```python
from build123d import *

# Parameters (mm, degrees)
BOSS_EXTRUDE1_DEPTH      = 10
BOSS_EXTRUDE1_DEPTH_BACK = 10
FILLET1_R                = 10


with BuildPart() as part:
    # Sketch1 → Boss-Extrude1 (new, two sides: drawn at the far end of the back side and taken through both)
    with BuildSketch(Plane.XY.offset(-BOSS_EXTRUDE1_DEPTH_BACK)):
        with BuildLine():
            Line((237.926881338, -1499.570637215), (237.926881338, -1519.570637215))
            Line((237.926881338, -1519.570637215), (214.725572022, -1519.570637215))
            ThreePointArc((214.725572022, -1519.570637215), (201.473903455, -1517.311772335), (189.718921324, -1510.790301224))
            Line((189.718921324, -1510.790301224), (-403.542618158, -1035.59351223))
            ThreePointArc((-403.542618158, -1035.59351223), (-414.593324739, -1021.690516088), (-418.53596746, -1004.37384822))
            Line((-418.53596746, -1004.37384822), (-418.53596746, -990.945694684))
            Line((-418.53596746, -990.945694684), (-398.53596746, -990.945694684))
            Line((-398.53596746, -990.945694684), (-398.53596746, -1004.37384822))
            ThreePointArc((-398.53596746, -1004.37384822), (-396.5646461, -1013.032182154), (-391.039292809, -1019.983680225))
            Line((-391.039292809, -1019.983680225), (202.222246673, -1495.180469219))
            ThreePointArc((202.222246673, -1495.180469219), (208.099737738, -1498.441204775), (214.725572022, -1499.570637215))
            Line((214.725572022, -1499.570637215), (237.926881338, -1499.570637215))
        make_face()
    extrude(amount=BOSS_EXTRUDE1_DEPTH + BOSS_EXTRUDE1_DEPTH_BACK)

    # Fillet1
    fillet1_edges = [part.edges().sort_by_distance(p)[0] for p in [
        (226.32622668, -1499.570637215, -10),
        (208.099737738, -1498.441204775, -10),
        (-398.53596746, -997.659771452, -10),
        (-396.5646461, -1013.032182154, -10),
        (-418.53596746, -997.659771452, -10),
        (-414.593324739, -1021.690516088, -10),
        (226.32622668, -1519.570637215, -10),
        (201.473903455, -1517.311772335, -10),
        (226.32622668, -1499.570637215, 10),
        (208.099737738, -1498.441204775, 10),
        (-398.53596746, -997.659771452, 10),
        (-396.5646461, -1013.032182154, 10),
        (-418.53596746, -997.659771452, 10),
        (-414.593324739, -1021.690516088, 10),
        (226.32622668, -1519.570637215, 10),
        (201.473903455, -1517.311772335, 10),
        (-94.408523068, -1257.582074722, -10),
        (-106.911848417, -1273.191906727, -10),
        (-94.408523068, -1257.582074722, 10),
        (-106.911848417, -1273.191906727, 10),
    ]]
    fillet(fillet1_edges, radius=FILLET1_R - 0.0001)  # a hair under: the kernel refuses the full size


solid = part.part
```
Can you work these out from the model? Positions are in its coordinate system, mm. Give positions to 0.01 mm unless a question says otherwise; leave off trailing zeros. Order: outer loops, then holes, each group sorted by start corner. A loop starts at its lowest first (then second) coordinate and runs counter-clockwise, first axis right, second up. Notation, with made-up numbers: M 33.5,83 L 90.5,83 A35 ccw 90.5,118 Z; hole C 85,31.25 d5. An arc over 180 degrees is marked long. One line per item, written item: value.
1) Please list where these lines run through material, in increasing order: line 1 along Z through (x, y) = (-283.5, -1117); line 2 along Y through (x, z) = (-215.5, -1); line 3 along Y through (x, z) = (-265, 0.75).
Answer sheet:
line 1: z = -9.89 to 9.89
line 2: y = -1186.15 to -1160.65
line 3: y = -1146.53 to -1120.98
2) I want a section at A-A, the plane z = 6.5. List the corners of the cut face in (x, y) for me, plus the area to 3 significant figures.
Answer sheet:
outline: M -416.14,-1004.37 A37.6 ccw -402.04,-1033.72 L 191.22,-1508.92 A37.6 ccw 214.73,-1517.17 L 237.93,-1517.17 L 237.93,-1501.97 L 214.73,-1501.97 A22.4 cw 200.72,-1497.05 L -392.54,-1021.86 A22.4 cw -400.94,-1004.37 L -400.94,-990.95 L -416.14,-990.95 Z
area: 12,800 mm^2
3) For P1, Ø3, axis at y = -1094.5, z = -0.5, coming from the -X side; P2, Ø4, axis at y = -1413.5, z = 7.5, coming from the -X side; P3, Ø3, axis at x = -250.5, z = -8, coming from the -Y side, each with a flat end and sliding along its axis, tell me the tip position at first contact or that it passes through.
Answer sheet:
P1: stops at x = -331.86
P2: stops at x = 69.79
P3: stops at y = -1155.48
